from build123d import *

# Parameters (mm, degrees)
SKETCH4_W           = 200
SKETCH4_H           = 125
BOSS_EXTRUDE2_DEPTH = 50
SKETCH6_W           = 75
SKETCH6_H           = 25
CUT_EXTRUDE1_DEPTH  = 201
SKETCH7_W           = 40
SKETCH7_H           = 50
CUT_EXTRUDE2_DEPTH  = 20
BOSS_EXTRUDE5_DEPTH = 40
SKETCH10_R          = 20
BOSS_EXTRUDE6_DEPTH = 50
BOSS_EXTRUDE8_DEPTH = 30


with BuildPart() as part:
    # Sketch4 → Boss-Extrude2 (new body)
    with BuildSketch(Plane(origin=(0, 0, 0), x_dir=(1, 0, 0), z_dir=(0, 1, 0))):
        with Locations((12.028985507, -7.427536232)):
            Rectangle(SKETCH4_W, SKETCH4_H)
    extrude(amount=BOSS_EXTRUDE2_DEPTH)

    # Sketch6 → Cut-Extrude1 (cut, through all)
    with BuildSketch(Plane.ZY.offset(87.971014493)):
        with Locations((7.427536232, 12.5)):
            Rectangle(SKETCH6_W, SKETCH6_H)
    extrude(amount=-CUT_EXTRUDE1_DEPTH, mode=Mode.SUBTRACT)

    # Sketch7 → Cut-Extrude2 (cut)
    with BuildSketch(Plane.XY.offset(69.927536232)):
        with Locations((12.028985507, 25)):
            Rectangle(SKETCH7_W, SKETCH7_H)
    extrude(amount=-CUT_EXTRUDE2_DEPTH, mode=Mode.SUBTRACT)

    # Sketch9 → Boss-Extrude5 (add)
    with BuildSketch(Plane.ZY.offset(-32.028985507)):
        Polygon((49.927536232, 50), (69.927536232, 0), (49.927536232, 0), align=None)
    extrude(amount=BOSS_EXTRUDE5_DEPTH)

    # Sketch10 → Boss-Extrude6 (add)
    with BuildSketch(Plane(origin=(0, 0, -55.072463768), x_dir=(-1, 0, 0), z_dir=(0, 0, -1))):
        with BuildLine():
            Line((-42.028985507, 50), (-112.028985507, 50))
            Line((-112.028985507, 50), (-112.028985507, 85))
            ThreePointArc((-112.028985507, 85), (-77.028985507, 120), (-42.028985507, 85))
            Line((-42.028985507, 85), (-42.028985507, 50))
        make_face()
        with Locations((-77.028985507, 85)):
            Circle(SKETCH10_R, mode=Mode.SUBTRACT)
    extrude(amount=-BOSS_EXTRUDE6_DEPTH)

    # Sketch11 → Boss-Extrude8 (add)
    with BuildSketch(Plane(origin=(0, 0, -55.072463768), x_dir=(-1, 0, 0), z_dir=(0, 0, -1))):
        with BuildLine():
            Line((-42.028985507, 50), (17.971014493, 50))
            Line((17.971014493, 50), (-52.905907859, 110.358965373))
            ThreePointArc((-52.905907859, 110.358965373), (-44.862949711, 98.796598898), (-42.028985507, 85))
            Line((-42.028985507, 85), (-42.028985507, 50))
        make_face()
    extrude(amount=-BOSS_EXTRUDE8_DEPTH)


solid = part.part
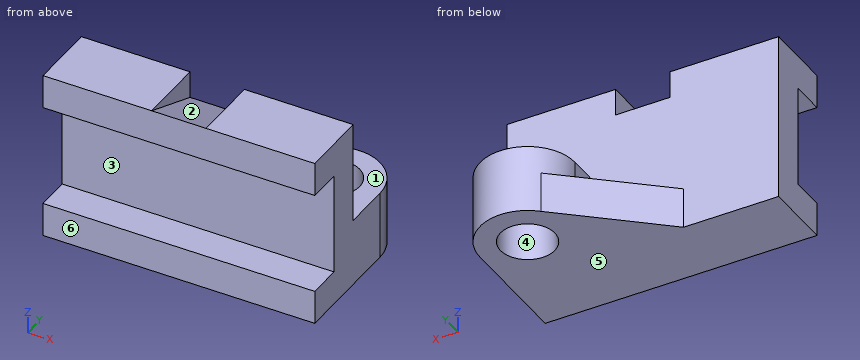
The listing builds one solid part. Answer for the finished solid, in the listing's coordinates (mm). Face numbers are marked on the shaded views. A direction names the side the tool comes from. Round coordinates to 2 decimals unless told otherwise and drop trailing zeros. Order: outer loops, then holes, each group sorted by start corner. A loop starts at its lowest first (then second) coordinate and runs counter-clockwise, first axis right, second up. Notation, with made-up numbers: (26, 3.5) -> (82, 3.5) arc R19 cw to (82, 40.5) -> close; hole circle Ø3 at (46, 24). An arc over 180 degrees is marked (long way). Write each question's results on one line, items separated by ' | '. Start each with the question number.
Q1. Each of these flat-tipped pins is pushed along its axis until it touches: pin 1 (10 mm diameter, centred on x = -32.5, z = 22.5, fed in from +Y); pin 2 (21 mm diameter, centred on x = 68.5, y = 89, fed in from +Z); pin 3 (6 mm diameter, centred on y = 62.5, z = -12.5, fed in from -X). Where does it stop, or does it pass through?
Q2. Straight lines are drawn through the part: probe 1 along Z at (x, y) = (54.5, 54); probe 2 along Y at (x, z) = (-58.5, -7); probe 3 along Z at (x, y) = (25, 78.5). For each, find the intervals that lie inside material, in ascending order. Write a range as from..to.
Q3. Find section D-D (z = 38). Determine the outline of the cut face in (x, y), then the cut area to 3 significant figures.
Q4. Find section C-C (x = -61). Determine the outline of the cut face in (y, z).
Q5. Which of the six approach directions +Z, -Z, +X, -X, +Y, -Y give full straight-line access (tool end or side, diameter ignored) to the marked faces 1, 2 and 3?
Q6. Find section A-A (y = 90). Determine the outline of the cut face in (x, z), then the cut area to 3 significant figures.
Q7. Find section B-B (z = -46). Determine the outline of the cut face in (x, y), then the cut area to 3 significant figures.
Q8. The mould has two halves that part along Y. Classify the marked faces 4, 5 and 6: pulls with the +Y half, pulls with the -Y half, needs draft (parallel to the pull), parting line crosses it, or undercut.
Worked answers:
1) pin 1: stops at y = 50 | pin 2: passes through | pin 3: stops at x = 42.03
2) probe 1: z = -55.07..-5.07 | probe 2: y = 25..50 | probe 3: z = -55.07..-25.07
3) outline: (-87.97, 25) -> (112.03, 25) -> (112.03, 50) -> (-87.97, 50) -> close | area: 5,000 mm2
4) outline: (0, -55.07) -> (50, -55.07) -> (50, 69.93) -> (0, 69.93) -> (0, 44.93) -> (25, 44.93) -> (25, -30.07) -> (0, -30.07) -> close
5) face 1: +Z, +X, -X, +Y | face 2: +Z, +Y | face 3: +X, -X, -Y
6) outline: (29, -55.07) -> (57.66, -55.07) -> (57.66, -5.07) -> (42.39, -5.07) -> (42.39, -25.07) -> (29, -25.07) -> close; (96.39, -55.07) -> (111.67, -55.07) -> (111.67, -5.07) -> (96.39, -5.07) -> close | area: 1,930 mm2
7) outline: (-87.97, 0) -> (112.03, 0) -> (112.03, 85) arc R35 ccw to (52.91, 110.36) -> (-17.97, 50) -> (-87.97, 50) -> close; hole circle Ø40 at (77.03, 85) | area: 14,700 mm2
8) face 4: undercut | face 5: needs draft | face 6: pulls with the -Y half
